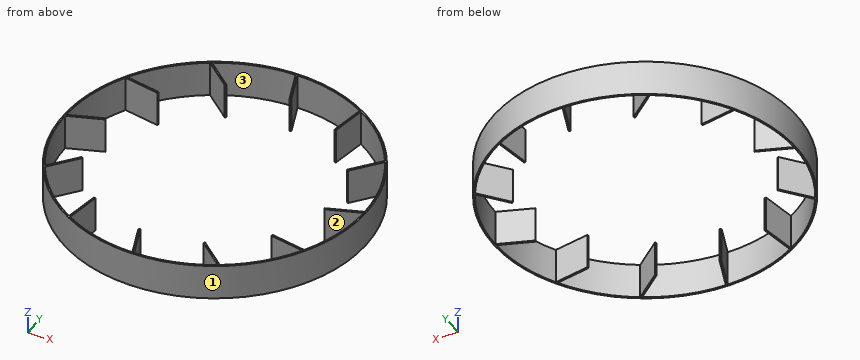
from build123d import *

# Parameters (mm, degrees)
SKETCH1_R           = 228.6
SKETCH1_R_2         = 226.06
BOSS_EXTRUDE1_DEPTH = 53.34
BOSS_EXTRUDE2_START = -53.34
BOSS_EXTRUDE2_DEPTH = 53.34


with BuildPart() as part:
    # Sketch1 → Boss-Extrude1 (new body)
    with BuildSketch(Plane.XY):
        Circle(SKETCH1_R)
        Circle(SKETCH1_R_2, mode=Mode.SUBTRACT)
    extrude(amount=BOSS_EXTRUDE1_DEPTH)

    # Sketch2 → Boss-Extrude2 (add)
    with BuildSketch(Plane.XY.offset(53.34).offset(BOSS_EXTRUDE2_START)):
        with BuildLine():
            Line((-226.06, 0), (-175.26, 18.123220102))
            Line((-175.26, 18.123220102), (-176.113474245, 20.515537328))
            Line((-176.113474245, 20.515537328), (-226.043844758, 2.702563026))
            ThreePointArc((-226.043844758, 2.702563026), (-226.055961153, 1.351305656), (-226.06, 0))
        make_face()
        with BuildLine():
            Line((-195.77370278, 113.03), (-142.718002216, 103.325169006))
            Line((-142.718002216, 103.325169006), (-142.260973981, 105.823713621))
            Line((-142.260973981, 105.823713621), (-194.408430417, 115.362410615))
            ThreePointArc((-194.408430417, 115.362410615), (-195.094552208, 114.198245603), (-195.77370278, 113.03))
        make_face()
        with BuildLine():
            Line((-113.03, 195.77370278), (-71.934830994, 160.841222318))
            Line((-71.934830994, 160.841222318), (-70.289760624, 162.776511309))
            Line((-70.289760624, 162.776511309), (-110.681434143, 197.110993443))
            ThreePointArc((-110.681434143, 197.110993443), (-111.857715551, 196.445857864), (-113.03, 195.77370278))
        make_face()
        with BuildLine():
            Line((0, 226.06), (18.123220102, 175.26))
            Line((18.123220102, 175.26), (20.515537328, 176.113474245))
            Line((20.515537328, 176.113474245), (2.702563026, 226.043844758))
            ThreePointArc((2.702563026, 226.043844758), (1.351305656, 226.055961153), (0, 226.06))
        make_face()
        with BuildLine():
            Line((113.03, 195.77370278), (103.325169006, 142.718002216))
            Line((103.325169006, 142.718002216), (105.823713621, 142.260973981))
            Line((105.823713621, 142.260973981), (115.362410615, 194.408430417))
            ThreePointArc((115.362410615, 194.408430417), (114.198245603, 195.094552208), (113.03, 195.77370278))
        make_face()
        with BuildLine():
            Line((195.77370278, 113.03), (160.841222318, 71.934830994))
            Line((160.841222318, 71.934830994), (162.776511309, 70.289760624))
            Line((162.776511309, 70.289760624), (197.110993443, 110.681434143))
            ThreePointArc((197.110993443, 110.681434143), (196.445857864, 111.857715551), (195.77370278, 113.03))
        make_face()
        with BuildLine():
            Line((226.06, 0), (175.26, -18.123220102))
            Line((175.26, -18.123220102), (176.113474245, -20.515537328))
            Line((176.113474245, -20.515537328), (226.043844758, -2.702563026))
            ThreePointArc((226.043844758, -2.702563026), (226.055961153, -1.351305656), (226.06, 0))
        make_face()
        with BuildLine():
            Line((195.77370278, -113.03), (142.718002216, -103.325169006))
            Line((142.718002216, -103.325169006), (142.260973981, -105.823713621))
            Line((142.260973981, -105.823713621), (194.408430417, -115.362410615))
            ThreePointArc((194.408430417, -115.362410615), (195.094552208, -114.198245603), (195.77370278, -113.03))
        make_face()
        with BuildLine():
            Line((113.03, -195.77370278), (71.934830994, -160.841222318))
            Line((71.934830994, -160.841222318), (70.289760624, -162.776511309))
            Line((70.289760624, -162.776511309), (110.681434143, -197.110993443))
            ThreePointArc((110.681434143, -197.110993443), (111.857715551, -196.445857864), (113.03, -195.77370278))
        make_face()
        with BuildLine():
            Line((0, -226.06), (-18.123220102, -175.26))
            Line((-18.123220102, -175.26), (-20.515537328, -176.113474245))
            Line((-20.515537328, -176.113474245), (-2.702563026, -226.043844758))
            ThreePointArc((-2.702563026, -226.043844758), (-1.351305656, -226.055961153), (0, -226.06))
        make_face()
        with BuildLine():
            Line((-113.03, -195.77370278), (-103.325169006, -142.718002216))
            Line((-103.325169006, -142.718002216), (-105.823713621, -142.260973981))
            Line((-105.823713621, -142.260973981), (-115.362410615, -194.408430417))
            ThreePointArc((-115.362410615, -194.408430417), (-114.198245603, -195.094552208), (-113.03, -195.77370278))
        make_face()
        with BuildLine():
            Line((-195.77370278, -113.03), (-160.841222318, -71.934830994))
            Line((-160.841222318, -71.934830994), (-162.776511309, -70.289760624))
            Line((-162.776511309, -70.289760624), (-197.110993443, -110.681434143))
            ThreePointArc((-197.110993443, -110.681434143), (-196.445857864, -111.857715551), (-195.77370278, -113.03))
        make_face()
    extrude(amount=BOSS_EXTRUDE2_DEPTH)


solid = part.part
Input: part model. Units: mm. Frame: model coordinates. Face numbers are marked on the shaded views. Give positions to 0.01 mm unless a question says otherwise; leave off trailing zeros. Write each loop counter-clockwise with the first axis right and the second up, starting at its lowest first coordinate (ties: lowest second). Pieces come first, ordered by that corner, then holes.
Q1. First-contact query: P1, Ø12, axis at x = 121.5, z = 6.5, coming from the -Y side; P2, Ø3, axis at y = 16.5, z = 25, coming from the +X side; P3, Ø2, axis at y = -36, z = 18.5, coming from the -X side. Flat tips, straight axial feed; report the tip coordinate or a pass-through.
Q2. Section B-B, the plane x = 91.5. Output: boundary loops of the cut face in (y, z).
Q3. Pull-direction query (Y, two-part tool) for the marked faces 1, 2 and 3; classes: pulls with the +Y half, pulls with the -Y half, needs draft (parallel to the pull), parting line crosses it, or undercut.
Q4. Section A-A, the plane x = 45.5. Output: boundary loops of the cut face in (y, z), plus the area to 3 significant figures.
Q5. Section C-C, the plane x = -36.5. Output: boundary loops of the cut face in (y, z), plus the area to 3 significant figures.
Q6. Material intervals for probe 1 along Y at (x, z) = (-71, 29.5); probe 2 along Y at (x, z) = (-79, 32); probe 3 along Y at (x, z) = (-168.5, 17.5), sorted ascending.
Filled in:
1. P1: stops at y = -197.28
1. P2: stops at x = 228.11
1. P3: stops at x = -225.9
2. outline: (-209.49, 0) - (-206.71, 0) - (-206.71, 53.34) - (-209.49, 53.34) - close; (-180.81, 0) - (-177.47, 0) - (-177.47, 53.34) - (-180.81, 53.34) - close; (206.71, 0) - (209.49, 0) - (209.49, 53.34) - (206.71, 53.34) - close
3. face 1: parting line crosses it
3. face 2: undercut
3. face 3: undercut
4. outline: (-224.03, 0) - (-221.43, 0) - (-221.43, 53.34) - (-224.03, 53.34) - close; (221.43, 0) - (224.03, 0) - (224.03, 53.34) - (221.43, 53.34) - close
4. area: 277 mm2
5. outline: (-225.67, 0) - (-223.09, 0) - (-223.09, 53.34) - (-225.67, 53.34) - close; (223.09, 0) - (225.67, 0) - (225.67, 53.34) - (223.09, 53.34) - close
5. area: 275 mm2
6. probe 1: y = -217.29 to -214.62, 161.94 to 163.38, 214.62 to 217.29
6. probe 2: y = -214.52 to -211.81, 166.85 to 170.18, 211.81 to 214.52
6. probe 3: y = -154.49 to -150.7, -80.94 to -77.02, 108.04 to 110.62, 150.7 to 154.49
